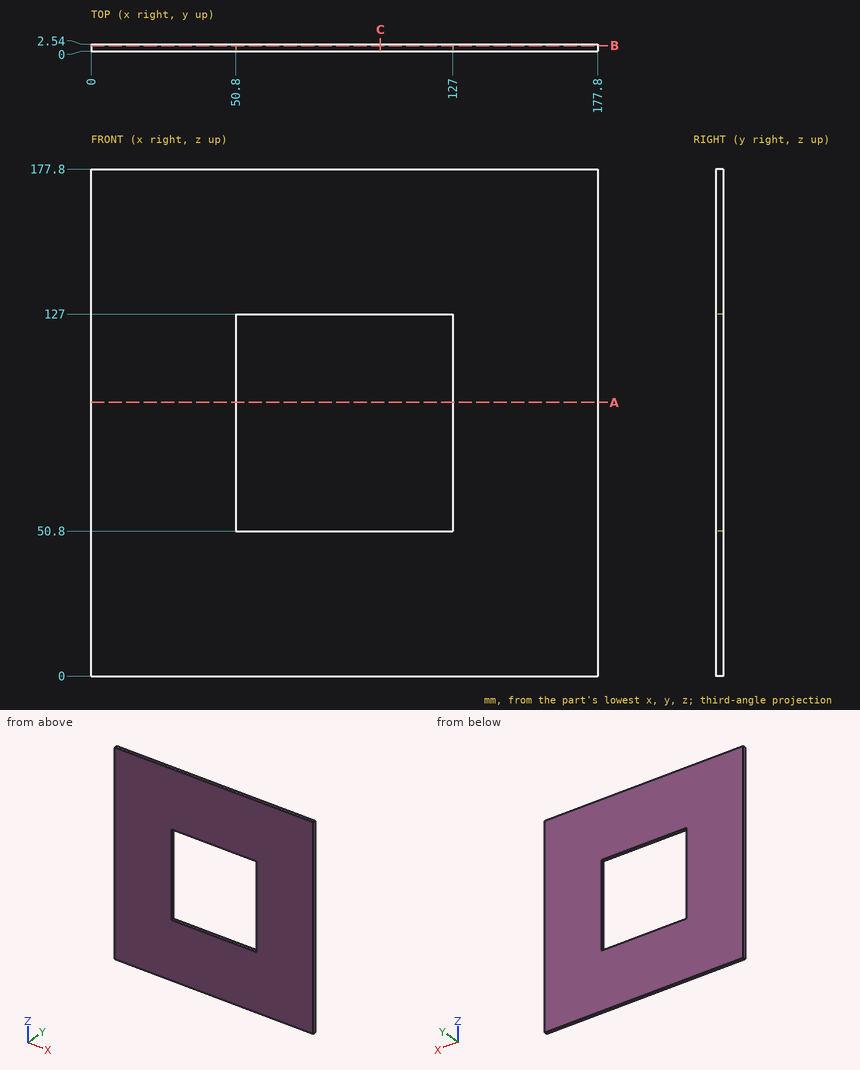
Study the drawing (mm; zero at the part's minimum x, y, z) and answer. Give positions to 0.01 mm unless a question says otherwise; leave off trailing zeros. Write each loop counter-clockwise with the first axis right and the second up, starting at its lowest first coordinate (ties: lowest second). Pieces come first, ordered by that corner, then holes. Notation, with made-up numbers: (10.25, 51) -> (64.25, 51) arc R34 cw to (64.25, 83) -> close; hole circle Ø10 at (-22.5, 30.25). An arc over 180 degrees is marked (long way). Answer in a Markdown table with one row per item.
1) A straight line is drawn through the part: line 1 (X direction, y = 1.15, z = 101.5). Find the intervals that lie inside material, in ascending order. Write a range as [from, to].
Results list:
| item | result |
|---|---|
| line 1 | [0, 50.8], [127, 177.8] |
2) Section A-A on z = 96 is taken. Give the vertices of the cut face in (x, y), plus the area to 3 significant figures.
Results list:
| item | result |
|---|---|
| outline | (0, 0) -> (50.8, 0) -> (50.8, 2.54) -> (0, 2.54) -> close; (127, 0) -> (177.8, 0) -> (177.8, 2.54) -> (127, 2.54) -> close |
| area | 258 mm^2 |
3) Section B-B on y = 1.95 is taken. Give the vertices of the cut face in (x, z).
Results list:
| item | result |
|---|---|
| outline | (0, 0) -> (177.8, 0) -> (177.8, 177.8) -> (0, 177.8) -> close; hole (50.8, 50.8) -> (127, 50.8) -> (127, 127) -> (50.8, 127) -> close |
4) Section C-C on x = 101.5 is taken. Give the vertices of the cut face in (y, z).
Results list:
| item | result |
|---|---|
| outline | (0, 0) -> (2.54, 0) -> (2.54, 50.8) -> (0, 50.8) -> close; (0, 127) -> (2.54, 127) -> (2.54, 177.8) -> (0, 177.8) -> close |
